from build123d import *

# Parameters (mm, degrees)
ESQUISSE1_R             = 1.5
BOSS_EXTRU_1_DEPTH      = 15.8
ESQUISSE2_R             = 9.01
ENL_V_MAT_EXTRU_1_DEPTH = 9.8
CHANFREIN1_SIZE         = 1
CONG_2_R                = 2


with BuildPart() as part:
    # Esquisse1 → Boss.-Extru.1 (new body)
    with BuildSketch(Plane.XY):
        with BuildLine():
            Line((1.732050808, 3), (20.767949192, 35.97114317))
            ThreePointArc((20.767949192, 35.97114317), (22.5, 36.97114317), (24.232050808, 35.97114317))
            Line((24.232050808, 35.97114317), (43.267949192, 3))
            ThreePointArc((43.267949192, 3), (43.267949192, 1), (41.535898385, 0))
            Line((41.535898385, 0), (3.464101615, 0))
            ThreePointArc((3.464101615, 0), (1.732050808, 1), (1.732050808, 3))
        make_face()
        with Locations((22.5, 31.97114317)):
            Circle(ESQUISSE1_R, mode=Mode.SUBTRACT)
        with Locations((38.937822174, 3.5)):
            Circle(ESQUISSE1_R, mode=Mode.SUBTRACT)
        with Locations(Location((6.062177826, 3.5, 0), (0, 0, 180))):
            Circle(ESQUISSE1_R, mode=Mode.SUBTRACT)
    extrude(amount=BOSS_EXTRU_1_DEPTH)

    # Esquisse2 → Enlèv. mat.-Extru.1 (cut)
    with BuildSketch(Plane(origin=(0, 0, 0), x_dir=(-1, 0, 0), z_dir=(0, 0, -1))):
        with Locations((-22.5, 12.990381057)):
            Circle(ESQUISSE2_R)
    extrude(amount=-ENL_V_MAT_EXTRU_1_DEPTH, mode=Mode.SUBTRACT)

    # Chanfrein1
    chanfrein1_edges = [part.edges().sort_by_distance(p)[0] for p in [
        (31.51, 12.990381057, 0),
    ]]
    chamfer(chanfrein1_edges, length=CHANFREIN1_SIZE)

    # Congé2
    cong_2_edges = [part.edges().sort_by_distance(p)[0] for p in [
        (43.267949192, 1, 15.8),
        (22.5, 0, 15.8),
        (1.732050808, 1, 15.8),
        (11.25, 19.485571585, 15.8),
        (22.5, 36.97114317, 15.8),
        (11.25, 19.485571585, 0),
        (1.732050808, 1, 0),
        (22.5, 0, 0),
        (43.267949192, 1, 0),
        (33.75, 19.485571585, 0),
        (22.5, 36.97114317, 0),
        (33.75, 19.485571585, 15.8),
    ]]
    fillet(cong_2_edges, radius=CONG_2_R - 0.0001)  # a hair under: the kernel refuses the full size


solid = part.part
The model under review builds one solid part; all positions refer to its coordinate system, in mm. A direction names the side the tool comes from. Coordinates: 2 decimals unless noted, no trailing zeros. Write each loop counter-clockwise with the first axis right and the second up, starting at its lowest first coordinate (ties: lowest second). Pieces come first, ordered by that corner, then holes. Notation, with made-up numbers: (-34, 10.5) -> (-13, 10.5) arc R17 cw to (-13, 22.5) -> close; hole circle Ø5 at (21, 19). An arc over 180 degrees is marked (long way). Answer in a Markdown table with one row per item.
1. We need section B-B, the plane y = 3.5. Give the number of separate pieces and of enclosed holes in the cut face, and give its area (3 significant figures).
Answers below:
| item | result |
|---|---|
| separate pieces | 3 |
| enclosed holes | 0 |
| area | 546 mm^2 |
2. We need section A-A, the plane z = 4.5. State the section outline as (x, y) points, and give its area (3 significant figures).
Answers below:
| item | result |
|---|---|
| outline | (1.73, 3) arc R2 ccw to (3.46, 0) -> (41.54, 0) arc R2 ccw to (43.27, 3) -> (24.23, 35.97) arc R2 ccw to (20.77, 35.97) -> close; hole circle Ø3 at (6.06, 3.5); hole circle Ø18.02 at (22.5, 12.99); hole circle Ø3 at (22.5, 31.97); hole circle Ø3 at (38.94, 3.5) |
| area | 592 mm^2 |
3. For faces 1 (the cylindrical face through (1.75, 0.97, 7.82)), 2 (the flat face through (23, 13, 9.8)), list the 3-axis set-ups (+Z, -Z, +X, -X, +Y, -Y) from which the entire face can be reached by the end or side of a thin tool; tool diameter is ignored.
Answers below:
| item | result |
|---|---|
| face 1 | +Z, -Z, -X |
| face 2 | -Z |
4. Clearance check with flat-ended pins moving along their axes: pin 1 Ø1 at (x, z) = (16.5, 9.5) entering from +Y; pin 2 Ø2 at (y, z) = (32.5, 3.5) entering from +X; pin 3 Ø2 at (x, z) = (38.5, 2.5) entering from +Y. State where each tip first meets the part, or that it passes through.
Answers below:
| item | result |
|---|---|
| pin 1 | stops at y = 29.44 |
| pin 2 | stops at x = 26.81 |
| pin 3 | stops at y = 12.99 |
5. Wall thickness on probe 1 along X at (y, z) = (32, 7.5); probe 2 along Y at (x, z) = (39, 5.5); probe 3 along Z at (x, y) = (21, 10): over which ranges is each line inside the solid? List them lowest first. Write a range as [from, to].
Answers below:
| item | result |
|---|---|
| probe 1 | x = [18.48, 21], [24, 26.52] |
| probe 2 | y = [0, 2], [5, 10.39] |
| probe 3 | z = [9.8, 15.8] |
